Part print with two shaded views. Sizes in mm from the minimum x, y, z corner. A direction names the side the tool comes from. Round coordinates to 2 decimals unless told otherwise and drop trailing zeros. Order: outer loops, then holes, each group sorted by start corner. A loop starts at its lowest first (then second) coordinate and runs counter-clockwise, first axis right, second up. Notation, with made-up numbers: (81, 83) -> (104, 83) arc R30 ccw to (104, 116) -> close; hole circle Ø2 at (-0.75, 48). An arc over 180 degrees is marked (long way). Answer as a JSON object with one key per item and string values.
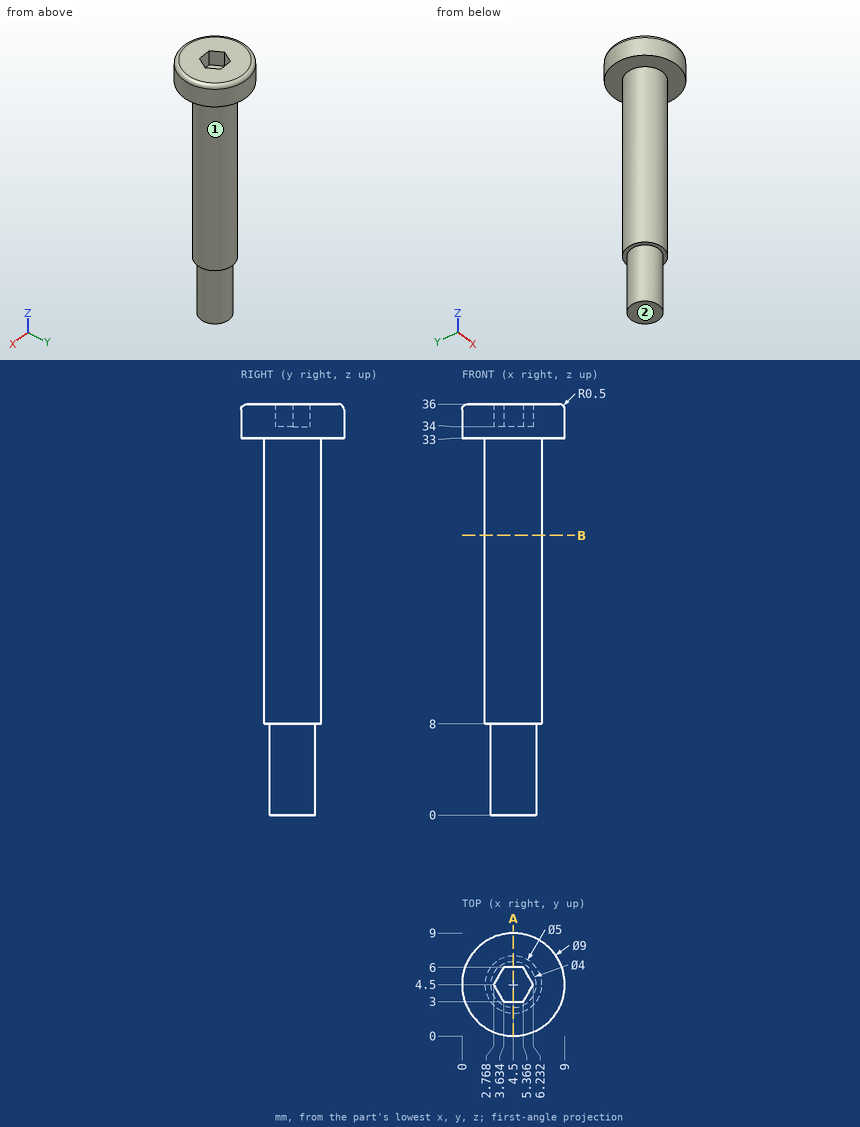
1) Cut at A-A, the plane x = 4.5. Give the cut face in (y, z), plus the area to 3 significant figures.
Checked values:
{"outline": "(0, 33) -> (2, 33) -> (2, 8) -> (2.5, 8) -> (2.5, 0) -> (6.5, 0) -> (6.5, 8) -> (7, 8) -> (7, 33) -> (9, 33) -> (9, 35.5) arc R0.5 ccw to (8.5, 36) -> (6, 36) -> (6, 34) -> (3, 34) -> (3, 36) -> (0.5, 36) arc R0.5 ccw to (0, 35.5) -> close", "area": "178 mm²"}
2) Probe L1, parallel to Z at x = 5, y = 5.25; L2, parallel to Y at x = 4.75, z = 34.5; L3, parallel to X at y = 6.5, z = 14. List the from-to ranges inside material, lowest first. Write a range as from..to.
Checked values:
{"L1": "z = 0..34", "L2": "y = 0.01..3, 6..8.99", "L3": "x = 3..6"}
3) Cut at B-B, the plane z = 24.5. Give the cut face in (x, y).
Checked values:
{"outline": "circle Ø5 at (4.5, 4.5)"}
4) Which spindle directions (+Z, -Z, +X, -X, +Y, -Y) get a long thin tool onto all of the face, cutting with end or side? Do the marked faces 1 and 2. Say none if no direction does.
Checked values:
{"face 1": "-Z", "face 2": "-Z, +X, -X, +Y, -Y"}
5) Flat gauge pins, fed straight in: pin 1 Ø2 at (y, z) = (4.5, 13) entering from -X; pin 2 Ø0.5 at (x, z) = (4, 35) entering from -Y; pin 3 Ø2 at (x, y) = (2, 7) entering from -Z. Where does each tip first touch, or does it go through?
Checked values:
{"pin 1": "stops at x = 2", "pin 2": "stops at y = 0.01", "pin 3": "stops at z = 33"}
